Check sheet for the drawn part. Datum: minimum x, y, z corner. Units: mm. Round coordinates to 2 decimals unless told otherwise and drop trailing zeros. Write each loop counter-clockwise with the first axis right and the second up, starting at its lowest first coordinate (ties: lowest second). Pieces come first, ordered by that corner, then holes.
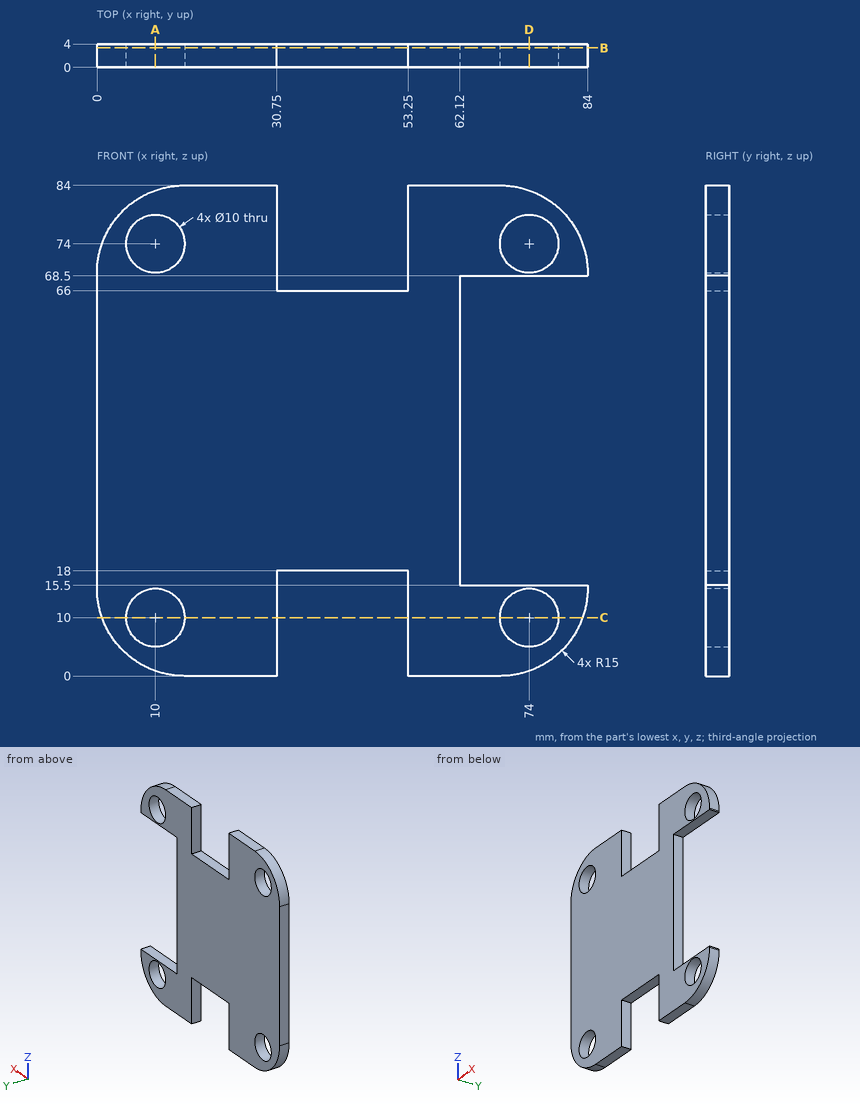
1. Sectioned sample at C-C, the plane z = 10. Enter the section's corners in (x, y), plus the area to 3 significant figures.
2. Go/stop test with flat-tipped pins: pin 1 (1 mm diameter, centred on y = 3, z = 22, fed in from +X); pin 2 (2 mm diameter, centred on x = 37.5, y = 1.5, fed in from -Z); pin 3 (1.2 mm diameter, centred on x = 72, y = 1.5, fed in from -Z); pin 4 (8 mm diameter, centred on x = 74, z = 74, fed in from +Y). Record where each tip stops, or that it passes through.
3. Scan lines: line 1 along X through (y, z) = (3.6, 75.5); line 2 along Z through (x, y) = (10, 2.6); line 3 along X through (y, z) = (1.1, 74). Record each from-to range of solid material in increasing order.
4. Sectioned sample at B-B, the plane y = 3.35. Enter the section's corners in (x, z).
5. Sectioned sample at A-A, the plane x = 10. Enter the section's corners in (y, z), plus the area to 3 significant figures.
6. Sectioned sample at D-D, the plane x = 74. Enter the section's corners in (y, z), plus the area to 3 significant figures.
Computed values:
1. outline: (0.86, 0) - (5, 0) - (5, 4) - (0.86, 4) - close; (15, 0) - (30.75, 0) - (30.75, 4) - (15, 4) - close; (53.25, 0) - (69, 0) - (69, 4) - (53.25, 4) - close; (79, 0) - (83.14, 0) - (83.14, 4) - (79, 4) - close
1. area: 159 mm2
2. pin 1: stops at x = 62.12
2. pin 2: stops at z = 18
2. pin 3: stops at z = 0.19
2. pin 4: passes through
3. line 1: x = 1.48 to 5.23, 14.77 to 30.75, 53.25 to 69.23, 78.77 to 82.52
3. line 2: z = 0.86 to 5, 15 to 69, 79 to 83.14
3. line 3: x = 0.86 to 5, 15 to 30.75, 53.25 to 69, 79 to 83.14
4. outline: (0, 15) arc R15 ccw to (15, 0) - (30.75, 0) - (30.75, 18) - (53.25, 18) - (53.25, 0) - (69, 0) arc R15 ccw to (84, 15) - (84, 15.5) - (62.12, 15.5) - (62.12, 68.5) - (84, 68.5) - (84, 69) arc R15 ccw to (69, 84) - (53.25, 84) - (53.25, 66) - (30.75, 66) - (30.75, 84) - (15, 84) arc R15 ccw to (0, 69) - close; hole circle Ø10 at (10, 10); hole circle Ø10 at (10, 74); hole circle Ø10 at (74, 10); hole circle Ø10 at (74, 74)
5. outline: (0, 0.86) - (4, 0.86) - (4, 5) - (0, 5) - close; (0, 15) - (4, 15) - (4, 69) - (0, 69) - close; (0, 79) - (4, 79) - (4, 83.14) - (0, 83.14) - close
5. area: 249 mm2
6. outline: (0, 0.86) - (4, 0.86) - (4, 5) - (0, 5) - close; (0, 15) - (4, 15) - (4, 15.5) - (0, 15.5) - close; (0, 68.5) - (4, 68.5) - (4, 69) - (0, 69) - close; (0, 79) - (4, 79) - (4, 83.14) - (0, 83.14) - close
6. area: 37.1 mm2
